Can you work these out from the model? Positions are in its coordinate system, mm. Round coordinates to 2 decimals unless told otherwise and drop trailing zeros. Order: outer loops, then holes, each group sorted by start corner. A loop starts at its lowest first (then second) coordinate and runs counter-clockwise, first axis right, second up.
Q1. If I drill on line 1 (Z direction, x = 32.5, y = -19); line 2 (Y direction, x = -14, z = 8.5); line 3 (Z direction, x = 40, y = -20.5), over which ranges is the centre line in solid material (lowest first)?
Q2. If we section it at B-B (z = 10.5): Please give me the cut outline in (x, y), plus the area to 3 significant figures.
Q3. If we section it at A-A (z = 1.5): Please give me the cut outline in (x, y).
Q4. Will these pins go through, and if not, where does the flat tip stop? P1, Ø0.7, axis at y = 1, z = -0.5, coming from the +X side; P2, Ø5, axis at x = -32.5, y = 18, coming from the -Z side; P3, Ø0.7, axis at y = 5.5, z = -0.5, coming from the -X side.
from build123d import *

# Parameters (mm, degrees)
F0_W     = 11.387274
F0_H     = 22.464488
F1_DEPTH = 12.7
F2_R     = 5.08
F3_DEPTH = 0.635


with BuildPart() as f1:
    # F0 (on Top) → F1 (new body)
    with BuildSketch(Plane.XY):
        with BuildLine():
            ThreePointArc((45.499377, 12.166495), (-46.696597, -6.135533), (47.09795, 0))
            ThreePointArc((47.09795, 0), (46.696597, 6.135533), (45.499377, 12.166495))
        make_face()
        with Locations((39.80574, 0.934251)):
            Rectangle(F0_W, F0_H, mode=Mode.SUBTRACT)
        with Locations((39.80574, 0.934251)):
            Rectangle(F0_W, F0_H)
    extrude(amount=F1_DEPTH)

    # F2
    f2_edges = [f1.edges().sort_by_distance(p)[0] for p in [
        (-47.09795, 0, 12.7),
    ]]
    fillet(f2_edges, radius=F2_R)

    # F0 (on Top) → F3 (join)
    with BuildSketch(Plane.XY):
        with Locations((39.80574, 0.934251)):
            Rectangle(F0_W, F0_H)
    extrude(amount=-F3_DEPTH)


solid = f1.part
Solution:
1. line 1: z = 0 to 12.7
1. line 2: y = -44.89 to 44.89
1. line 3: z = 0 to 11.77
2. outline: (44.63, 11.94) arc R46.2 ccw (long way) to (46.2, 0) arc R46.2 ccw to start
2. area: 6,710 mm2
3. outline: (45.5, 12.17) arc R47.1 ccw (long way) to (47.1, 0) arc R47.1 ccw to start
4. P1: stops at x = 45.5
4. P2: stops at z = 0
4. P3: stops at x = 34.11
